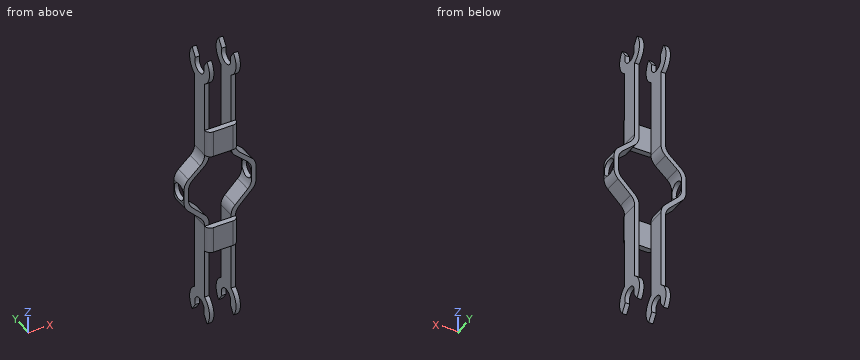
Autodesk Inventor part; units mm, degrees
ref_plane "YZ Plane" through (0, 0, 0) normal (1, 0, 0) x (0, 1, 0)
ref_plane "XZ Plane" through (0, 0, 0) normal (0, 1, 0) x (-1, 0, 0)
ref_plane "XY Plane" through (0, 0, 0) normal (0, 0, 1) x (1, 0, 0)
sketch "Sketch1" plane through (0, 0, 0) normal (0, 1, 0) x (-1, 0, 0)
  line L0 (-1.778, -22.923) -> (-1.778, 0)
  line L1 (-0.508, -7.6359) -> (-0.508, -7.8464)
  line L2 (0, -7.62) -> (2.3608, -9.743)
  line L3 (-0.508, -7.8464) -> (1.8528, -9.9694)
  line L4 (2.3608, -10.0755) -> (2.3608, -9.743)
  line L5 (1.8528, -9.9694) -> (1.8528, -12.5094)
  line L6 (2.3608, -12.7283) -> (2.3608, -10.0755)
  line L7 (1.8528, -12.5094) -> (-0.508, -14.8702)
  line L8 (2.3608, -12.7283) -> (0, -15.1057)
  line L9 (-0.508, -15.1057) -> (-0.508, -25.2657)
  line L10 (-0.508, -25.2657) -> (0, -25.2657)
  line L11 (0, -25.2657) -> (0, -15.1057)
  line L12 (-0.508, -15.1057) -> (-0.508, -14.8702)
  line L13 (-0.508, -7.6359) -> (-0.508, 2.5241)
  line L14 (-0.508, 2.5241) -> (0, 2.5241)
  line L15 (0, 2.5241) -> (0, -7.62)
  line L16 (-5.4088, -9.9694) -> (-5.4088, -12.5094)
  line L17 (-5.9168, -12.7283) -> (-5.9168, -10.0755)
  line L18 (-3.048, -15.1057) -> (-3.048, -14.8702)
  line L19 (-5.4088, -12.5094) -> (-3.048, -14.8702)
  line L20 (-5.9168, -12.7283) -> (-3.556, -15.1057)
  line L21 (-3.048, -15.1057) -> (-3.048, -25.2657)
  line L22 (-3.048, -25.2657) -> (-3.556, -25.2657)
  line L23 (-3.556, -25.2657) -> (-3.556, -15.1057)
  line L24 (-5.9168, -10.0755) -> (-5.9168, -9.743)
  line L25 (-3.048, -7.8464) -> (-5.4088, -9.9694)
  line L26 (-3.556, -7.62) -> (-5.9168, -9.743)
  line L27 (-3.048, -7.6359) -> (-3.048, -7.8464)
  line L28 (-3.048, 2.5241) -> (-3.556, 2.5241)
  line L29 (-3.556, 2.5241) -> (-3.556, -7.62)
  line L30 (-3.048, -7.6359) -> (-3.048, 2.5241)
  point P0 (2.5714, -13.0979)
  point P1 (-0.508, -7.6086)
  point P2 (-6.1274, -13.0979)
  point P3 (-3.048, -7.6086)
extrude "Extrusion1" add sketch "Sketch1" along normal blind 2.032
sketch "Sketch3" plane through (0, 0, 0) normal (0, -1, 0) x (1, 0, 0)
  line L0 (3.556, 0) -> (3.556, -6.9126)
  line L1 (0, -6.9126) -> (3.556, -6.9126)
  line L2 (3.556, -6.9126) -> (3.556, -3.8646)
  line L3 (3.556, -3.8646) -> (0, -3.8646)
  line L4 (0, -3.8646) -> (0, -6.9126)
  line L5 (0, -22.923) -> (0, -15.76)
  line L6 (3.556, -15.76) -> (3.556, -22.923)
  line L7 (0, -15.76) -> (3.556, -15.76)
  line L8 (3.556, -15.76) -> (3.556, -18.808)
  line L9 (3.556, -18.808) -> (0, -18.808)
  line L10 (0, -18.808) -> (0, -15.76)
  point P0 (0, 0)
  dimension "d33" = 3.048
  dimension "d34" = 3.048
extrude "Extrusion3" add sketch "Sketch3" along normal blind 0.635
fillet "Fillet4" radius 0.635 4 edges at (3.556, -0.635, -5.3886) (0, -0.635, -5.3886) (0, -0.635, -17.284) (3.556, -0.635, -17.284)
sketch "Sketch6" plane through (3.048, 0, -3.8646) normal (0, 0, 1) x (1, 0, 0)
  line L0 (-2.54, 2.032) -> (-0.0025, 2.032)
  line L1 (-0.0025, 2.032) -> (-0.0025, -3.9837)
  line L2 (-0.0025, -3.9837) -> (-2.54, -3.9837)
  line L3 (-2.54, -3.9837) -> (-2.54, 2.032)
  line L4 (-0.0025, -3.9837) -> (-2.54, -3.9837)
  line L5 (-2.54, -3.9837) -> (-2.54, 4.1191)
  line L6 (-2.54, 4.1191) -> (-0.0025, 4.1191)
  line L7 (-0.0025, 4.1191) -> (-0.0025, -3.9837)
  point P0 (-3.048, 0)
extrude "Extrusion6" cut sketch "Sketch6" along normal through all
sketch "Sketch9" plane through (0.508, 0, -18.808) normal (0, 0, -1) x (-1, 0, 0)
  line L0 (0, 0) -> (0.508, 0)
  line L1 (0, 0) -> (-2.54, 0)
  line L2 (-2.54, 0) -> (-2.54, 7.62)
  line L3 (-2.54, 7.62) -> (0, 7.62)
  line L4 (0, 7.62) -> (0, 0)
  line L5 (-2.54, 7.62) -> (0, 7.62)
  line L6 (0, 7.62) -> (0, -7.6202)
  line L7 (0, -7.6202) -> (-2.54, -7.6202)
  line L8 (-2.54, -7.6202) -> (-2.54, 7.62)
  dimension "d50" = 2.54
  dimension "d51" = 7.62
extrude "Extrusion8" cut sketch "Sketch9" along normal through all
fillet "Fillet6" radius 1.524 16 edges at (5.9168, 1.016, -9.743) (3.556, 1.016, -7.62) (3.048, 1.016, -7.8464) (5.4088, 1.016, -9.9694) (5.4088, 1.016, -12.5094) (5.9168, 1.016, -12.7283) (3.048, 1.016, -14.8702) (3.556, 1.016, -15.1057) (-2.3608, 1.016, -12.7283) (0, 1.016, -15.1057) (0.508, 1.016, -14.8702) (-1.8528, 1.016, -12.5094) (-2.3608, 1.016, -9.743) (-1.8528, 1.016, -9.9694) (0, 1.016, -7.62) (0.508, 1.016, -7.8464)
sketch "Sketch11" plane through (0, 0, -25.2657) normal (-1, 0, 0) x (0, 0, 1)
  arc A0 (-2.3402, -0.4747) -> (-2.3402, 2.5067) centre (-1.016, 1.016) ccw
  line L0 (-1.016, 0.0802) -> (0.5328, 0.0802) construction
  line L1 (-1.016, 1.9518) -> (0.5328, 1.9518) construction
  arc A1 (-2.3402, -0.4747) -> (-2.3402, 2.5067) centre (-1.016, 1.016) ccw
  arc A2 (-1.4219, 0.1684) -> (-1.4219, 1.8636) centre (-1.016, 1.016) ccw
  line L2 (-1.4219, 1.8636) -> (-2.3402, 2.5067)
  line L3 (-1.4219, 1.8636) -> (-0.3008, 1.8636) construction
  line L4 (-1.4219, 0.1684) -> (-2.3402, -0.4747)
  line L5 (-1.4219, 0.1684) -> (-0.3008, 0.1684) construction
  point P0 (25.2657, 0)
  dimension "d66" = 3.9878
  dimension "d74" = 1.8796
  dimension "d75" = 145
  dimension "d76" = 145
extrude "Extrusion10" add sketch "Sketch11" against normal blind 3.556
sketch "Sketch12" plane through (3.048, 0, -18.808) normal (0, 0, -1) x (-1, 0, 0)
  line L0 (0, -7.62) -> (2.54, -7.62)
  line L1 (2.54, -7.62) -> (2.54, 11.139)
  line L2 (2.54, 11.139) -> (0, 11.139)
  line L3 (0, 11.139) -> (0, -7.62)
  point P0 (3.048, 0)
extrude "Extrusion11" cut sketch "Sketch12" along normal through all
ref_plane "Work Plane3" through (3.048, 0, -11.3322) normal (0, 0, -1) x (-1, 0, 0)
mirror "Mirror2" about plane through (3.048, 0, -11.3322) normal (0, 0, -1) of "Extrusion10"
mirror "Mirror3" about plane through (3.048, 0, -11.3322) normal (0, 0, -1) of "Extrusion11"
sketch "Sketch13" plane through (5.9168, 0, -10.4221) normal (1, 0, 0) x (0, 0, -1)
  circle A0 centre (0.8382, 1.016) radius 0.9525
  point P0 (-10.4221, 0)
  dimension "d77" = 1.905
extrude "Extrusion12" cut sketch "Sketch13" against normal through all
properties part number "rocker" material "Aluminum 6061"
Model file for the job. Use its own axes, mm. Coordinates: 2 decimals unless noted, no trailing zeros. Loops run counter-clockwise (first coordinate to the right, second up) from the corner with the lowest first, then second, coordinate; pieces in that order, holes last. Notation, with made-up numbers: (-31.5, 40.25) - (7.5, 40.25) arc R31 cw to (7.5, 74.25) - close; hole circle Ø10 at (51.5, -27.75). An arc over 180 degrees is marked (long way). Write item = value, one per line. Start each with the question number.
Item 1: Wall check: probe 1 along X at (y, z) = (0.15, -24); probe 2 along Z at (x, y) = (-0.5, 0.2); probe 3 along X at (y, z) = (1.05, -13). Give the ranges that are in metal, low to high. Write a range as [from, to].
Item 2: Saw through at B-B, the plane x = 1.75. List the corners of the cut face in (y, z) (3 decimals).
Item 3: Saw through at A-A, the plane z = -22.5. List the corners of the cut face in (x, y), then the cut area to 3 significant figures.
Item 4: Drop flat-ended pins along their axis: pin 1 Ø2 at (y, z) = (2, -20.5) entering from +X; pin 2 Ø0.7 at (x, y) = (1.5, -0.5) entering from +Z; pin 3 Ø0.9 at (x, z) = (-1.5, -12) entering from -Y. Give the stop position or say it passes through.
Item 5: Saw through at C-C, the plane z = -5. List the corners of the cut face in (x, y) (3 decimals).
Answers:
q1.probe_1 = [0, 0.51], [3.05, 3.56]
q1.probe_2 = [-14.6, -13.86], [-8.75, -8.07]
q1.probe_3 = [-2.07, -1.36], [4.92, 5.62]
q2.outline = (-0.635, -18.808) - (0, -18.808) - (0, -15.76) - (-0.635, -15.76) - close; (-0.635, -6.913) - (0, -6.913) - (0, -3.865) - (-0.635, -3.865) - close
q3.outline = (0, 0) - (0.51, 0) - (0.51, 2.03) - (0, 2.03) - close; (3.05, 0) - (3.56, 0) - (3.56, 2.03) - (3.05, 2.03) - close
q3.area = 2.06 mm2
q4.pin_1 = 3.56
q4.pin_2 = -3.86
q4.pin_3 = 0
q5.outline = (0, 0) arc R0.635 ccw to (0.635, -0.635) - (2.921, -0.635) arc R0.635 ccw to (3.556, 0) - (3.556, 2.032) - (3.048, 2.032) - (3.048, 0) - (0.508, 0) - (0.508, 2.032) - (0, 2.032) - close
